The figure shows three views and two pictorial views of one solid part (mm, origin at its lowest corner). Answer the questions. Give positions to 0.01 mm unless a question says otherwise; leave off trailing zeros. Write each loop counter-clockwise with the first axis right and the second up, starting at its lowest first coordinate (ties: lowest second). Pieces come first, ordered by that corner, then holes. Notation, with made-up numbers: M 12.5,20.5 L 28.5,20.5 A21 ccw 28.5,29.5 Z; hole C 18.5,-30 d10. An arc over 180 degrees is marked long. Return JSON: item names as keys, results as strings.
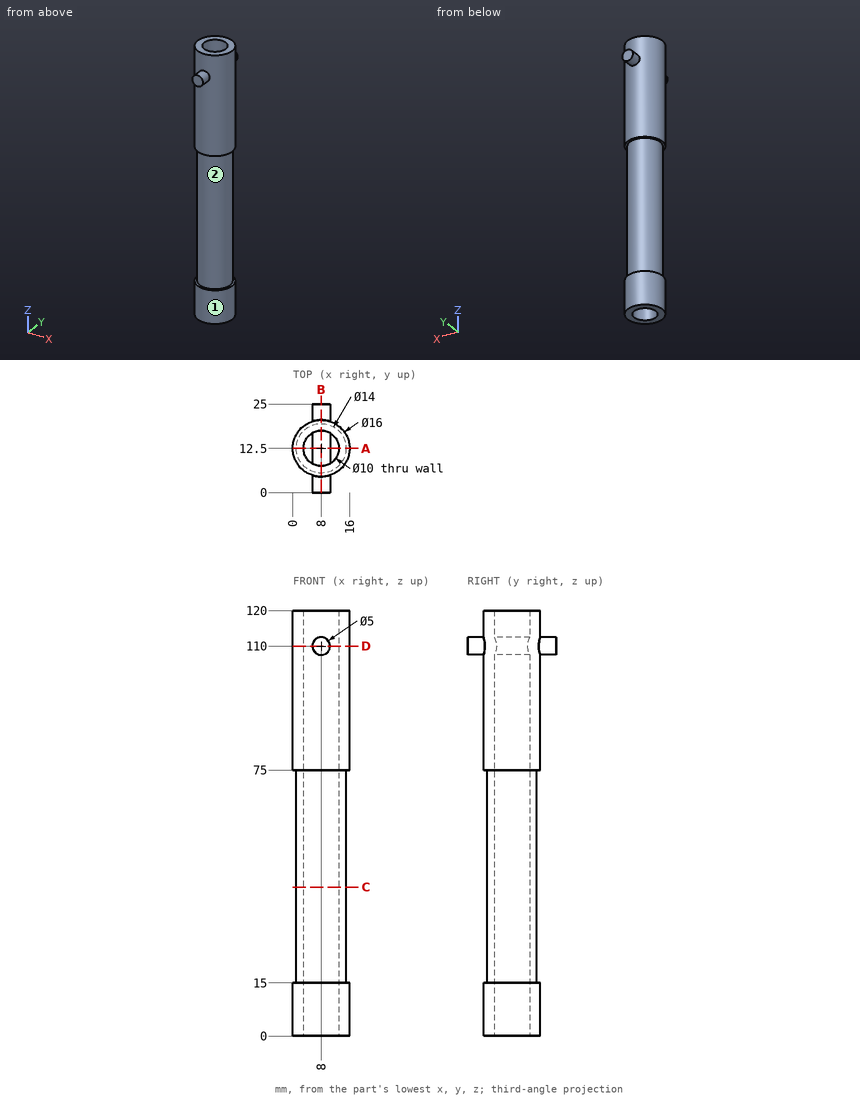
Item 1: A cutting plane is placed at C-C, the plane z = 42. Write down the section's boundary in (x, y).
Geometry results:
{"outline": "C 8,12.5 d14; hole C 8,12.5 d10"}
Item 2: Find the intervals of material crossed by line 1 (Y direction, x = 8, z = 79.5); line 2 (Y direction, x = 8, z = 74.5); line 3 (X direction, y = 9, z = 11), in increasing order.
Geometry results:
{"line 1": "y = 4.5 to 7.5, 17.5 to 20.5", "line 2": "y = 5.5 to 7.5, 17.5 to 19.5", "line 3": "x = 0.81 to 4.43, 11.57 to 15.19"}
Item 3: Determine the mould class of the marked faces 1 and 2 for opening direction Z: +Z half, -Z half, draft (parallel to the pull), parting line (faces both ways), or undercut.
Geometry results:
{"face 1": "draft", "face 2": "undercut"}
Item 4: A cutting plane is placed at D-D, the plane z = 110. Write down the section's boundary in (x, y).
Geometry results:
{"outline": "M 5.5,0 L 10.5,0 L 10.5,4.9 A8 ccw 10.5,20.1 L 10.5,25 L 5.5,25 L 5.5,20.1 A8 ccw 5.5,4.9 Z; hole M 5.5,8.17 L 5.5,16.83 A5 ccw Z; hole M 10.5,8.17 A5 ccw 10.5,16.83 Z"}
Item 5: A cutting plane is placed at A-A, the plane y = 12.5. Write down the section's boundary in (x, z), plus the area to 3 significant figures.
Geometry results:
{"outline": "M 0,0 L 3,0 L 3,120 L 0,120 L 0,75 L 1,75 L 1,15 L 0,15 Z; C 8,110 d5; M 13,0 L 16,0 L 16,15 L 15,15 L 15,75 L 16,75 L 16,120 L 13,120 Z", "area": "620 mm2"}
Item 6: A cutting plane is placed at B-B, the plane x = 8. Write down the section's boundary in (y, z), plus the area to 3 significant figures.
Geometry results:
{"outline": "M 0,107.5 L 4.5,107.5 L 4.5,75 L 5.5,75 L 5.5,15 L 4.5,15 L 4.5,0 L 7.5,0 L 7.5,107.5 L 17.5,107.5 L 17.5,0 L 20.5,0 L 20.5,15 L 19.5,15 L 19.5,75 L 20.5,75 L 20.5,107.5 L 25,107.5 L 25,112.5 L 20.5,112.5 L 20.5,120 L 17.5,120 L 17.5,112.5 L 7.5,112.5 L 7.5,120 L 4.5,120 L 4.5,112.5 L 0,112.5 Z", "area": "695 mm2"}
Item 7: Given pin 1 Ø1 at (x, z) = (4, 69) entering from +Y; pin 2 Ø3 at (x, z) = (5, 71) entering from +Y; pin 3 Ø3 at (x, z) = (10, 73) entering from -Y; pin 4 Ø4 at (x, y) = (11.5, 13.5) entering from -Z, each flat-ended and moving along its own axis, determine where each tip first touches the part or whether it passes through.
Geometry results:
{"pin 1": "stops at y = 18.56", "pin 2": "stops at y = 19.34", "pin 3": "stops at y = 5.52", "pin 4": "stops at z = 0"}
